The listing builds one solid part. Answer for the finished solid, in the listing's coordinates (mm). A direction names the side the tool comes from. Coordinates: 2 decimals unless noted, no trailing zeros. Order: outer loops, then holes, each group sorted by start corner. A loop starts at its lowest first (then second) coordinate and runs counter-clockwise, first axis right, second up. Notation, with made-up numbers: (0, 0) -> (16, 0) arc R23 cw to (16, 16) -> close; hole circle Ø6 at (20.25, -5.5). An arc over 180 degrees is marked (long way). Put each result on its own line as item: value. Start each with the question number.
```python
from build123d import *

# Parameters (mm, degrees)
SKETCH2_W           = 12.7
SKETCH2_H           = 13.8176
BOSS_EXTRUDE1_DEPTH = 6.35
SKETCH4_R           = 1.1938
CUT_EXTRUDE1_DEPTH  = 20.812586145
CUT_EXTRUDE2_DEPTH  = 20.812586145
SKETCH8_R           = 1.4605
CUT_EXTRUDE3_DEPTH  = 20.812586145
SKETCH9_R           = 2.7813
CUT_EXTRUDE4_DEPTH  = 20.442799947


with BuildPart() as part:
    # Sketch2 → Boss-Extrude1 (new body)
    with BuildSketch(Plane.XY):
        with Locations((6.35, 6.9088)):
            Rectangle(SKETCH2_W, SKETCH2_H)
    extrude(amount=BOSS_EXTRUDE1_DEPTH)

    # Sketch4 → Cut-Extrude1 (cut, through all)
    with BuildSketch(Plane(origin=(12.7, 0, 0), x_dir=(0, 0, -1), z_dir=(1, 0, 0))):
        with Locations((-2.3876, 2.3876)):
            Circle(SKETCH4_R)
        with BuildLine():
            Line((0, 2.3876), (2.839420075, 2.3876))
            Line((2.839420075, 2.3876), (2.839420075, -2.482839526))
            Line((2.839420075, -2.482839526), (-2.3876, -2.482839526))
            Line((-2.3876, -2.482839526), (-2.3876, 0))
            ThreePointArc((-2.3876, 0), (-0.699311849, 0.699311849), (0, 2.3876))
        make_face()
    extrude(amount=-CUT_EXTRUDE1_DEPTH, mode=Mode.SUBTRACT)

    # Sketch7 → Cut-Extrude2 (cut, through all)
    with BuildSketch(Plane(origin=(12.7, 0, 0), x_dir=(0, 0, -1), z_dir=(1, 0, 0))):
        Polygon((0, 2.3876), (-1.031425935, 14.176852388), (1.156682431, 14.176852388), (1.156682431, 2.3876), align=None)
    extrude(amount=-CUT_EXTRUDE2_DEPTH, mode=Mode.SUBTRACT)

    # Sketch8 → Cut-Extrude3 (cut, through all)
    with BuildSketch(Plane.XY.offset(6.35)):
        with Locations((3.175, 10.6426)):
            Circle(SKETCH8_R)
        with Locations(Location((9.525, 10.6426, 0), (0, 0, 90))):
            Circle(SKETCH8_R)
    extrude(amount=-CUT_EXTRUDE3_DEPTH, mode=Mode.SUBTRACT)

    # Sketch9 → Cut-Extrude4 (cut, through all)
    with BuildSketch(Plane.XY.offset(1.27)):
        with Locations((3.175, 10.6426)):
            Circle(SKETCH9_R)
        with Locations((9.525, 10.6426)):
            Circle(SKETCH9_R)
    extrude(amount=-CUT_EXTRUDE4_DEPTH, mode=Mode.SUBTRACT)


solid = part.part
```
(1) The part is cut by section D-D on y = 11. Determine the outline of the cut face in (x, z), plus the area to 3 significant figures.
(2) Find the intervals of material crossed by L1, parallel to Y at x = 4.5, z = 3; L2, parallel to X at y = 11.25, z = 5; L3, parallel to Y at x = 9.75, z = 1.75, in increasing order.
(3) The part is cut by section B-B on z = 2.75. Determine the outline of the cut face in (x, y) (1 decimal), plus the area to 3 significant figures.
(4) A tool of negligible diameter and unlimited length cuts with its end or side. For faces 1 (the cylindrical face through (2.98, 12.09, 3.85)), 2 (the cylindrical face through (8.922, 7.927, 0.949)), from which of +Z, -Z, +X, -X, +Y, -Y can it reach the whole face along a straight path? Write none if from no direction.
(5) For a pull along X with two mould halves and no side action, classify faces 3 (the flat face through (0, 7, 3)), 4 (the cylindrical face through (2.572, 7.927, 0.949)), 5 (the flat face through (6, 7, 6.35)) as released by +X, released by -X, zero draft, split by the parting line, or undercut.
(6) The part is cut by section A-A on x = 2.75. Determine the outline of the cut face in (y, z).
(7) Each of these flat-tipped pins is pushed along its axis until it touches: P1, Ø6, axis at x = 2, y = 12, coming from the -Z side; P2, Ø7, axis at x = 3.18, y = 10.64, coming from the -Z side; P3, Ø3, axis at x = 8, y = 7, coming from the -Z side. Where does it stop, or does it pass through?
(8) The part is cut by section C-C on y = 1.5. Determine the outline of the cut face in (x, z).
Worked out:
1. outline: (0, 0.75) -> (0.42, 0.75) -> (0.42, 1.27) -> (1.76, 1.27) -> (1.76, 6.35) -> (0, 6.35) -> close; (4.59, 1.27) -> (5.93, 1.27) -> (5.93, 0.75) -> (6.77, 0.75) -> (6.77, 1.27) -> (8.11, 1.27) -> (8.11, 6.35) -> (4.59, 6.35) -> close; (10.94, 1.27) -> (12.28, 1.27) -> (12.28, 0.75) -> (12.7, 0.75) -> (12.7, 6.35) -> (10.94, 6.35) -> close
1. area: 36.6 mm2
2. L1: 0 to 1.36, 3.41 to 10.03, 11.26 to 13.82
2. L2: 0 to 1.85, 4.5 to 8.2, 10.85 to 12.7
2. L3: 0.09 to 1.38, 3.4 to 9.2, 12.09 to 13.82
3. outline: (0, 0) -> (12.7, 0) -> (12.7, 1.3) -> (0, 1.3) -> close; (0, 3.5) -> (12.7, 3.5) -> (12.7, 13.8) -> (0, 13.8) -> close; hole circle Ø2.9 at (3.2, 10.6); hole circle Ø2.9 at (9.5, 10.6)
3. area: 133 mm2
4. face 1: +Z, -Z
4. face 2: -Z
5. face 3: released by -X
5. face 4: undercut
5. face 5: zero draft
6. outline: (0, 2.39) arc R2.39 ccw to (2.39, 0) -> (7.89, 0.48) -> (7.89, 1.27) -> (9.25, 1.27) -> (9.25, 6.35) -> (0, 6.35) -> close; (12.04, 1.27) -> (13.39, 1.27) -> (13.39, 0.96) -> (13.82, 1) -> (13.82, 6.35) -> (12.04, 6.35) -> close; hole circle Ø2.39 at (2.39, 2.39)
7. P1: z = 0.6
7. P2: z = 0.42
7. P3: z = 0.27
8. outline: (0, 0.17) -> (12.7, 0.17) -> (12.7, 1.59) -> (0, 1.59) -> close; (0, 3.19) -> (12.7, 3.19) -> (12.7, 6.35) -> (0, 6.35) -> close
